Geometry: final body of the model. Coordinates: model frame, mm. A direction names the side the tool comes from. Round coordinates to 2 decimals unless told otherwise and drop trailing zeros. Write each loop counter-clockwise with the first axis right and the second up, starting at its lowest first coordinate (ties: lowest second). Pieces come first, ordered by that corner, then holes. Notation, with made-up numbers: (70.25, 18.25) -> (84.25, 18.25) arc R18 cw to (84.25, 34.25) -> close; hole circle Ø7 at (55, 72.25). An arc over 180 degrees is marked (long way). Use one line per item in the form item = value. Start each with the question number.
1. Reachability of faces 4 (the face through (79, 54, 0)), 5 (the face through (31.277, 119.444, -1.565)), 6 (the face through (78, 56, -3.175)) from +Z, -Z, +X, -X, +Y, -Y: full face, straight path, thin tool, end or side. Return the list, or none.
2. Cut plane A-A, the plane y = 104. Return the cut outline in (x, z) (3 decimals).
3. Line query: L1, parallel to Y at x = 55, z = -1.5; L2, parallel to X at y = 72.5, z = -5.5 (3 decimals); L3, parallel to X at y = 82, z = -1. Output: solid intervals per line, ascending.
4. Cut plane B-B, the plane z = -8.5. Return the cut outline in (x, y) (3 decimals), plus the area to 3 significant figures.
5. Draft query along Y for faces 1 (the face through (123.825, 88, -8)), 2 (the face through (97.346, 50, -2)), 3 (the face through (64, 38.1, -3)). Return one class per face: pulls with the +Y half, pulls with the -Y half, needs draft (parallel to the pull), parting line crosses it, or undercut.
6. Cut plane D-D, the plane x = 63.5. Return the cut outline in (y, z) (1 decimal), plus the area to 3 significant figures.
7. Cut plane C-C, the plane x = 87. Return the cut outline in (y, z) (3 decimals).
```python
from build123d import *

# Parameters (mm, degrees)
BOSS_EXTRUDE1_DEPTH     = 139.7
SKETCH3_W               = 118.872
SKETCH3_H               = 40.64
SKETCH3_W_2             = 127
SKETCH3_H_2             = 38.1
CUT_EXTRUDE1_DEPTH      = 10.525
CUT_EXTRUDE1_DEPTH_BACK = 4.175
FILLET1_R               = 2.2352
CUT_EXTRUDE2_DEPTH      = 13.7


with BuildPart() as part:
    # Sketch2 → Boss-Extrude1 (new body)
    with BuildSketch(Plane(origin=(0, 0, 0), x_dir=(1, 0, 0), z_dir=(0, 1, 0))):
        Polygon((0, 0), (0, 12.7), (3.175, 12.7), (3.175, 3.175), (123.825, 3.175), (123.825, 12.7), (127, 12.7), (127, 0), align=None)
    extrude(amount=BOSS_EXTRUDE1_DEPTH)

    # Sketch3 → Cut-Extrude1 (cut, two sides)
    with BuildSketch(Plane(origin=(0, 0, -3.175), x_dir=(-1, 0, 0), z_dir=(0, 0, -1))) as cut_extrude1_sk:
        with BuildLine():
            Line((-6.35, 110.49), (-120.65, 110.49))
            ThreePointArc((-120.65, 110.49), (-122.936, 112.776), (-120.65, 115.062))
            Line((-120.65, 115.062), (-6.35, 115.062))
            ThreePointArc((-6.35, 115.062), (-4.064, 112.776), (-6.35, 110.49))
        make_face()
        with BuildLine():
            Line((-6.35, 62.738), (-120.65, 62.738))
            ThreePointArc((-120.65, 62.738), (-122.936, 65.024), (-120.65, 67.31))
            Line((-120.65, 67.31), (-6.35, 67.31))
            ThreePointArc((-6.35, 67.31), (-4.064, 65.024), (-6.35, 62.738))
        make_face()
        with Locations((-63.5, 88.9)):
            Rectangle(SKETCH3_W, SKETCH3_H)
        with Locations((-63.5, 19.05)):
            Rectangle(SKETCH3_W_2, SKETCH3_H_2)
    extrude(amount=CUT_EXTRUDE1_DEPTH, mode=Mode.SUBTRACT)
    extrude(cut_extrude1_sk.sketch, amount=-CUT_EXTRUDE1_DEPTH_BACK, mode=Mode.SUBTRACT)

    # Fillet1
    fillet1_edges = [part.edges().sort_by_distance(p)[0] for p in [
        (4.064, 68.58, -1.5875),
        (122.936, 68.58, -1.5875),
        (122.936, 109.22, -1.5875),
        (4.064, 109.22, -1.5875),
    ]]
    fillet(fillet1_edges, radius=FILLET1_R)

    # Sketch4 → Cut-Extrude2 (cut, through all)
    with BuildSketch(Plane.XY):
        with BuildLine():
            Line((32.8295, 133.731), (32.8295, 121.031))
            ThreePointArc((32.8295, 121.031), (31.242, 119.4435), (29.6545, 121.031))
            Line((29.6545, 121.031), (29.6545, 133.731))
            ThreePointArc((29.6545, 133.731), (31.242, 135.3185), (32.8295, 133.731))
        make_face()
        with BuildLine():
            Line((32.8295, 56.769), (32.8295, 44.069))
            ThreePointArc((32.8295, 44.069), (31.242, 42.4815), (29.6545, 44.069))
            Line((29.6545, 44.069), (29.6545, 56.769))
            ThreePointArc((29.6545, 56.769), (31.242, 58.3565), (32.8295, 56.769))
        make_face()
        with BuildLine():
            Line((61.9125, 133.731), (61.9125, 121.031))
            ThreePointArc((61.9125, 121.031), (63.5, 119.4435), (65.0875, 121.031))
            Line((65.0875, 121.031), (65.0875, 133.731))
            ThreePointArc((65.0875, 133.731), (63.5, 135.3185), (61.9125, 133.731))
        make_face()
        with BuildLine():
            Line((61.9125, 56.769), (61.9125, 44.069))
            ThreePointArc((61.9125, 44.069), (63.5, 42.4815), (65.0875, 44.069))
            Line((65.0875, 44.069), (65.0875, 56.769))
            ThreePointArc((65.0875, 56.769), (63.5, 58.3565), (61.9125, 56.769))
        make_face()
        with BuildLine():
            Line((94.1705, 133.731), (94.1705, 121.031))
            ThreePointArc((94.1705, 121.031), (95.758, 119.4435), (97.3455, 121.031))
            Line((97.3455, 121.031), (97.3455, 133.731))
            ThreePointArc((97.3455, 133.731), (95.758, 135.3185), (94.1705, 133.731))
        make_face()
        with BuildLine():
            Line((94.1705, 56.769), (94.1705, 44.069))
            ThreePointArc((94.1705, 44.069), (95.758, 42.4815), (97.3455, 44.069))
            Line((97.3455, 44.069), (97.3455, 56.769))
            ThreePointArc((97.3455, 56.769), (95.758, 58.3565), (94.1705, 56.769))
        make_face()
    extrude(amount=-CUT_EXTRUDE2_DEPTH, mode=Mode.SUBTRACT)


solid = part.part
```
Outcome:
q1.face_4 = +Z, +X, -X, +Y, -Y
q1.face_5 = +Z, -Z
q1.face_6 = -Z, +Y, -Y
q2.outline = (0, -12.7) -> (3.175, -12.7) -> (3.175, -3.175) -> (4.064, -3.175) -> (4.064, 0) -> (0, 0) -> close; (122.936, -3.175) -> (123.825, -3.175) -> (123.825, -12.7) -> (127, -12.7) -> (127, 0) -> (122.936, 0) -> close
q3.L1 = 38.1 to 62.74, 67.31 to 68.58, 109.22 to 110.49, 115.06 to 139.7
q3.L2 = 0 to 3.175, 123.825 to 127
q3.L3 = 0 to 4.06, 122.94 to 127
q4.outline = (0, 38.1) -> (3.175, 38.1) -> (3.175, 139.7) -> (0, 139.7) -> close; (123.825, 38.1) -> (127, 38.1) -> (127, 139.7) -> (123.825, 139.7) -> close
q4.area = 645 mm^2
q5.face_1 = needs draft
q5.face_2 = undercut
q5.face_3 = pulls with the -Y half
q6.outline = (38.1, -3.2) -> (42.5, -3.2) -> (42.5, 0) -> (38.1, 0) -> close; (58.4, -3.2) -> (62.7, -3.2) -> (62.7, 0) -> (58.4, 0) -> close; (67.3, -3.2) -> (68.6, -3.2) -> (68.6, 0) -> (67.3, 0) -> close; (109.2, -3.2) -> (110.5, -3.2) -> (110.5, 0) -> (109.2, 0) -> close; (115.1, -3.2) -> (119.4, -3.2) -> (119.4, 0) -> (115.1, 0) -> close; (135.3, -3.2) -> (139.7, -3.2) -> (139.7, 0) -> (135.3, 0) -> close
q6.area = 63.7 mm^2
q7.outline = (38.1, -3.175) -> (62.738, -3.175) -> (62.738, 0) -> (38.1, 0) -> close; (67.31, -3.175) -> (68.58, -3.175) -> (68.58, 0) -> (67.31, 0) -> close; (109.22, -3.175) -> (110.49, -3.175) -> (110.49, 0) -> (109.22, 0) -> close; (115.062, -3.175) -> (139.7, -3.175) -> (139.7, 0) -> (115.062, 0) -> close
